Verification items for the finished model (mm, model axes). A direction names the side the tool comes from. Round coordinates to 2 decimals unless told otherwise and drop trailing zeros. Order: outer loops, then holes, each group sorted by start corner. A loop starts at its lowest first (then second) coordinate and runs counter-clockwise, first axis right, second up. Notation, with made-up numbers: M 12,-18.75 L 54,-18.75 A21 ccw 54,-12.75 Z; hole C 10.25,-33 d11. An arc over 180 degrees is marked long. Return JSON: item names as keys, results as strings. Group by question number.
Autodesk Inventor part; units mm, degrees
ref_plane "YZ Plane" through (0, 0, 0) normal (1, 0, 0) x (0, 1, 0)
ref_plane "XZ Plane" through (0, 0, 0) normal (0, 1, 0) x (-1, 0, 0)
ref_plane "XY Plane" through (0, 0, 0) normal (0, 0, 1) x (1, 0, 0)
sketch "Sketch1" plane through (0, 0, 0) normal (1, 0, 0) x (0, 1, 0)
  circle A0 centre (0, 0) radius 14.2875
  dimension "d0" = 28.575
extrude "Extrusion1" add sketch "Sketch1" along normal blind 7.9248
sketch "Sketch2" plane through (7.9248, 0, 0) normal (1, 0, 0) x (0, 0, -1)
  point P0 (0, 0)
sketch "Sketch3" plane through (7.9248, 0, 0) normal (1, 0, 0) x (0, 0, -1)
  point P0 (0, 0)
sketch "Sketch4" plane through (7.9248, 0, 0) normal (1, 0, 0) x (0, 0, -1)
  line L0 (7.978, 4.7625) -> (8.1134, -4.5279)
  line L1 (8.1134, -4.5279) -> (0.1355, -9.2904)
  line L2 (0.1355, -9.2904) -> (-7.978, -4.7625)
  line L3 (-7.978, -4.7625) -> (-8.1134, 4.5279)
  line L4 (-8.1134, 4.5279) -> (-0.1355, 9.2904)
  line L5 (-0.1355, 9.2904) -> (7.978, 4.7625)
  point P0 (0, 0)
  point P1 (0, 0)
  dimension "d3" = 9.525
  dimension "d4" = 18.5807
extrude "Extrusion2" cut sketch "Sketch4" against normal blind 279.4
sketch "Sketch5" plane through (7.9248, 0, 0) normal (1, 0, 0) x (0, 0, -1)
  circle A0 centre (0, 0) radius 15.875
  dimension "d7" = 31.75
extrude "Extrusion3" add sketch "Sketch5" against normal blind 1.6002
extrude "Extrusion4" cut sketch "Sketch4" against normal blind 1.6002
extrude "Extrusion5" add sketch "Sketch4" against normal blind 2.54
extrude "Extrusion6" cut sketch "Sketch4" against normal blind 2.54
properties part number "hexagon bearing"
1. Cross-section at C-C (z = 6). Enter the section's corners in (x, y).
2. Cross-section at D-D (y = -12). Enter the section's corners in (x, z), plus the area to 3 significant figures.
3. Access from +Z, -Z, +X, -X, +Y, -Y to the whole of each face (thin tool, end or side, straight path). Record for faces 4 (the face through (4.018, 6.876, 4.18)), 5 (the face through (7.925, 7.3, 3.8)).
4. Go/stop test with flat-tipped pins: pin 1 (4 mm diameter, centred on x = 6.5, y = -12, fed in from -Z); pin 2 (1.5 mm diameter, centred on x = 3.5, z = -9.5, fed in from +Y); pin 3 (4 mm diameter, centred on y = 12, z = 9.5, fed in from -X); pin 4 (8 mm diameter, centred on y = -2.5, z = 0, fed in from +X). Record where each tip stops, or that it passes through.
5. Cross-section at A-A (x = 3.75). Enter the section's corners in (y, z) (1 decimal), plus the area to 3 significant figures.
6. Thickness scan on line 1 along Z through (x, y) = (5.25, -7.5); line 2 along Z through (x, y) = (5.25, 5); line 3 along Y through (x, z) = (1.5, -2). Record the ranges inside material, lowest first. Write a range as from..to.
7. Cross-section at B-B (y = 0). Enter the section's corners in (x, z) (1 decimal), plus the area to 3 significant figures.
8. Draft check along Y on faces 1 (the face through (4.02, -7.06, 3.86)), 2 (the face through (3.118, -14.274, -0.628)), 3 (the face through (6.325, 8.31, 11.83)). Enter one of: +Y half, -Y half, draft (parallel to the pull), parting line (faces both ways), or undercut.
Computed:
{
 "1": {"outline": "M 0,-12.97 L 6.32,-12.97 L 6.32,-14.7 L 7.92,-14.7 L 7.92,-5.87 L 0,-5.87 Z; M 0,5.79 L 7.92,5.79 L 7.92,14.7 L 6.32,14.7 L 6.32,12.97 L 0,12.97 Z"},
 "2": {"outline": "M 0,-7.75 L 6.32,-7.75 L 6.32,-10.39 L 7.92,-10.39 L 7.92,10.39 L 6.32,10.39 L 6.32,7.75 L 0,7.75 Z", "area": "131 mm²"},
 "3": {"face 4": "+X, -X", "face 5": "+Z, -Z, +X, +Y, -Y"},
 "4": {"pin 1": "stops at z = -12.33", "pin 2": "stops at y = 11.29", "pin 3": "stops at x = 0", "pin 4": "passes through"},
 "5": {"outline": "C 0,0 d28.6; hole M -9.3,-0.1 L -4.5,-8.1 L 4.8,-8 L 9.3,0.1 L 4.5,8.1 L -4.8,8 Z", "area": "417 mm²"},
 "6": {"line 1": "z = -12.16..-3.13, 3.07..12.16", "line 2": "z = -13.38..-7.55, 7.32..13.38", "line 3": "y = -14.15..-8.18, 8.1..14.15"},
 "7": {"outline": "M 0,-14.3 L 6.3,-14.3 L 6.3,-15.9 L 7.9,-15.9 L 7.9,-8 L 0,-8 Z; M 0,8 L 7.9,8 L 7.9,15.9 L 6.3,15.9 L 6.3,14.3 L 0,14.3 Z", "area": "104 mm²"},
 "8": {"face 1": "undercut", "face 2": "parting line", "face 3": "draft"}
}
